from build123d import *

# Parameters (mm, degrees)
SKETCH_1_W          = 145
SKETCH_1_H          = 54.239140964
SKETCH_1_R          = 15
EXTRUDE_1_DEPTH     = 14
CUT_EXTRUDE_1_DEPTH = 50
FILLET_2_R          = 5
SKETCH_3_R          = 2.5
CUT_EXTRUDE_2_DEPTH = 36
SKETCH_4_W          = 40.34248958
SKETCH_4_H          = 54.239140964
SKETCH_4_R          = 15
EXTRUDE_2_DEPTH     = 16


with BuildPart() as part:
    # Эскиз1 → Вытянуть1 (new body)
    with BuildSketch(Plane(origin=(0, 0, 0), x_dir=(1, 0, 0), z_dir=(0, 1, 0))):
        with Locations((52.5, 0)):
            Rectangle(SKETCH_1_W, SKETCH_1_H)
        with Locations(Location((0, 0, 0), (0, 0, 270))):
            Circle(SKETCH_1_R, mode=Mode.SUBTRACT)
    extrude(amount=EXTRUDE_1_DEPTH)

    # Эскиз2 → Вырез-Вытянуть1 (cut)
    with BuildSketch(Plane(origin=(0, 0, 0), x_dir=(1, 0, 0), z_dir=(0, 1, 0))):
        with BuildLine():
            Line((93.569014329, -10), (130.542559867, -10))
            Line((130.542559867, -10), (130.542559867, 10))
            Line((130.542559867, 10), (93.573862666, 10))
            ThreePointArc((93.573862666, 10), (90.74600698, 8.828998449), (89.573862992, 6.001616112))
            Line((89.573862992, 6.001616112), (89.569014656, -5.998383888))
            ThreePointArc((89.569014656, -5.998383888), (90.74001588, -8.827855685), (93.569014329, -10))
        make_face()
    extrude(amount=CUT_EXTRUDE_1_DEPTH, mode=Mode.SUBTRACT)

    # Скругление2
    fillet_2_edges = [part.edges().sort_by_distance(p)[0] for p in [
        (125, 7, 10),
        (125, 7, -10),
        (125, 7, 27.119570482),
        (125, 7, -27.119570482),
    ]]
    fillet(fillet_2_edges, radius=FILLET_2_R)

    # Эскиз3 → Вырез-Вытянуть2 (cut, symmetric)
    with BuildSketch(Plane.XY):
        with Locations(Location((107.871367235, 7.461129595, 0), (0, 0, 180))):
            Circle(SKETCH_3_R)
    extrude(amount=CUT_EXTRUDE_2_DEPTH, both=True, mode=Mode.SUBTRACT)

    # Эскиз4 → Вытянуть2 (add)
    with BuildSketch(Plane(origin=(0, 14, 0), x_dir=(1, 0, 0), z_dir=(0, 1, 0))):
        with Locations((0.17124479, 0)):
            Rectangle(SKETCH_4_W, SKETCH_4_H)
        with Locations(Location((0, 0, 0), (0, 0, 270))):
            Circle(SKETCH_4_R, mode=Mode.SUBTRACT)
    extrude(amount=EXTRUDE_2_DEPTH)


solid = part.part
Build history of the part. All positions in model axes, mm. A direction names the side the tool comes from. Coordinates: 2 decimals unless noted, no trailing zeros. Order: outer loops, then holes, each group sorted by start corner. A loop starts at its lowest first (then second) coordinate and runs counter-clockwise, first axis right, second up. Notation, with made-up numbers: (-13.75, 74) - (36.25, 74) arc R16 ccw to (36.25, 87) - close; hole circle Ø10 at (60, -10). An arc over 180 degrees is marked (long way). Write each question's results on one line, items separated by ' | '. Start each with the question number.
Item 1: Band-saw the part on C-C on y = 3.5. Write the cut outline in (x, z).
Item 2: Wall check: probe 1 along X at (y, z) = (10, 0); probe 2 along Z at (x, y) = (102, 9); probe 3 along X at (y, z) = (14.75, 0). Give the ranges that are in metal, low to high. Write a range as [from, to].
Item 3: Band-saw the part on D-D on z = -2.5. Write the cut outline in (x, y).
Item 4: Band-saw the part on B-B on z = -18. Write the cut outline in (x, y), and give its area (3 significant figures).
Item 5: Tool access for faces 1 (the face through (20.342, 22, 0)), 2 (the face through (104, 7, 10)), 3 (the face through (123.5, 7.1, -25.69)): list every direction of +Z, -Z, +X, -X, +Y, -Y with a clear straight run to the whole face (end or side of a thin tool).
Item 6: Mould opens along Z. For faces 4 (the face through (105.487, 6.71, 18.68)), 5 (the face through (33, 11, -27.12)), 6 (the face through (90.71, 6.9, 8.8)) say: released by +Z, released by -Z, zero draft, split by the parting line, or undercut.
Item 7: Flat gauge pins, fed straight in: pin 1 (17.5 mm diameter, centred on y = 21.5, z = 3.5, fed in from +X); pin 2 (10 mm diameter, centred on y = 24, z = 2, fed in from +X); pin 3 (3 mm diameter, centred on x = 32.5, z = -15, fed in from +Y). Where does each tip first touch, or does it go through?
Item 8: Band-saw the part on A-A on x = -9. Write the cut outline in (y, z), and give its area (3 significant figures).
Numbers:
1) outline: (-20, -27.12) - (120, -27.12) arc R5 ccw to (125, -22.12) - (125, -15) arc R5 ccw to (120, -10) - (93.57, -10) arc R4 cw to (89.57, -6) - (89.57, 6) arc R4 cw to (93.57, 10) - (120, 10) arc R5 ccw to (125, 15) - (125, 22.12) arc R5 ccw to (120, 27.12) - (-20, 27.12) - close; hole circle Ø30 at (0, 0)
2) probe 1: [-20, -15], [15, 89.57] | probe 2: [-27.12, -10], [10, 27.12] | probe 3: [-20, -15], [15, 20.34]
3) outline: (-20, 0) - (-14.79, 0) - (-14.79, 30) - (-20, 30) - close; (14.79, 0) - (89.57, 0) - (89.57, 14) - (20.34, 14) - (20.34, 30) - (14.79, 30) - close
4) outline: (-20, 0) - (125, 0) - (125, 14) - (20.34, 14) - (20.34, 30) - (-20, 30) - close; hole circle Ø5 at (107.87, 7.46) | area: 2,660 mm^2
5) face 1: +Z, -Z, +X, +Y | face 2: +X, +Y, -Y | face 3: -Z, +X, +Y, -Y
6) face 4: zero draft | face 5: released by -Z | face 6: undercut
7) pin 1: x = 90.11 | pin 2: x = 20.34 | pin 3: y = 14
8) outline: (0, -27.12) - (30, -27.12) - (30, -12) - (0, -12) - close; (0, 12) - (30, 12) - (30, 27.12) - (0, 27.12) - close | area: 907 mm^2
